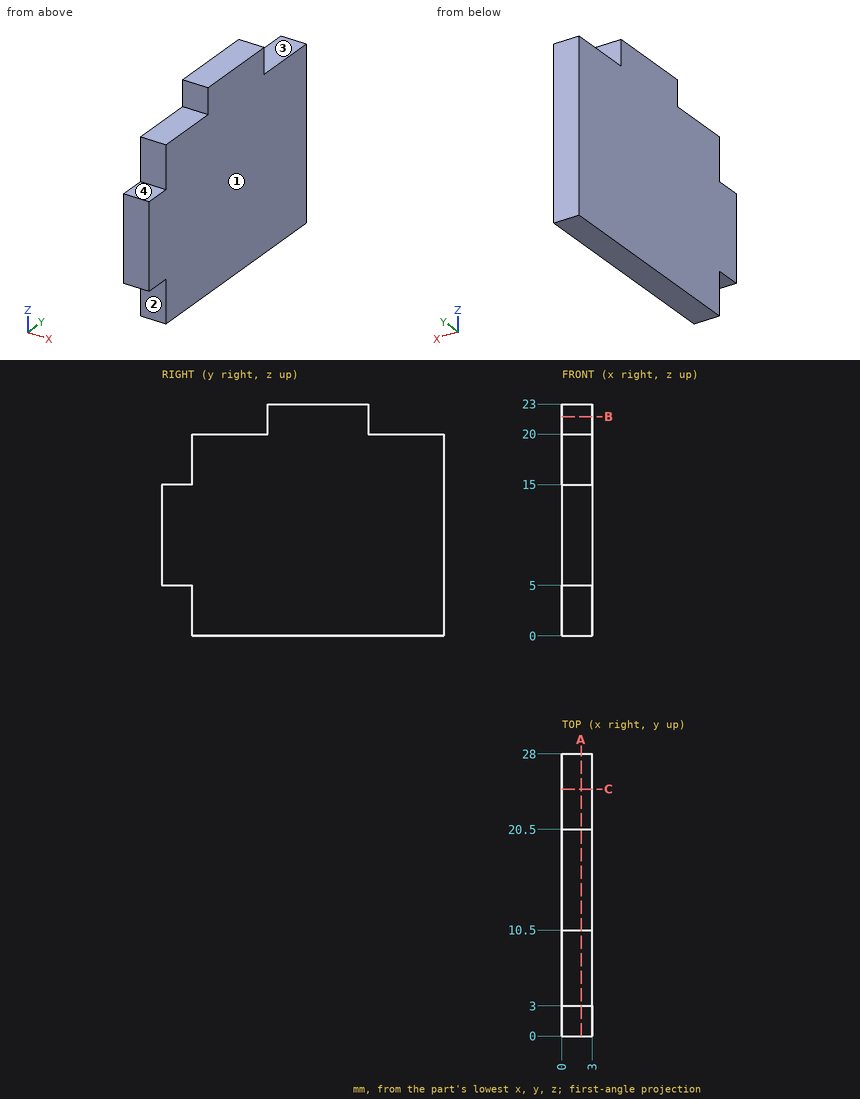
Can you work these out from the drawing? Everything is in mm from the part's minimum corner. A direction names the side the tool comes from. Round coordinates to 2 decimals unless told otherwise and drop trailing zeros. Loops run counter-clockwise (first coordinate to the right, second up) from the corner with the lowest first, then second, coordinate; pieces in that order, holes last. Notation, with made-up numbers: (23.25, 68) - (49.25, 68) arc R25 cw to (49.25, 92) - close; hole circle Ø6 at (56.5, -22.75). An arc over 180 degrees is marked (long way). Answer in a Markdown table with one row per item. Add a question column.
(1) I'm going to push flat-ended pins straight in: pin 1 (1 mm diameter, centred on x = 2, y = 18.5, fed in from -Z); pin 2 (0.9 mm diameter, centred on x = 1.5, z = 22, fed in from -Y); pin 3 (1.5 mm diameter, centred on x = 1.5, y = 1.5, fed in from -Z); pin 4 (1.5 mm diameter, centred on x = 1, z = 1.5, fed in from -Y). Where does each tip first touch, or does it pass through?
(2) If we section it at A-A (x = 1.9): Please give me the cut outline in (y, z).
(3) For the marked faces 1, 2, 3 and 4, which set-ups out of +Z, -Z, +X, -X, +Y, -Y let a thin tool reach every point of the face, with its end or its side?
(4) If we section it at C-C (y = 24.5): Please give me the cut outline in (x, z), plus the area to 3 significant figures.
(5) I need wall thicknesses on line 1 along Z through (x, y) = (1.7, 4.5); line 2 along Z through (x, y) = (1.1, 2.5); line 3 along Y through (x, z) = (2.2, 4.5). Which ranges of each line are inside material? Lowest first, please.
(6) If we section it at B-B (z = 21.75): Please give me the cut outline in (x, y), plus the area to 3 significant figures.
Model answer:
| question | item | result |
|---|---|---|
| 1 | pin 1 | stops at z = 0 |
| 1 | pin 2 | stops at y = 10.5 |
| 1 | pin 3 | stops at z = 5 |
| 1 | pin 4 | stops at y = 3 |
| 2 | outline | (0, 5) - (3, 5) - (3, 0) - (28, 0) - (28, 20) - (20.5, 20) - (20.5, 23) - (10.5, 23) - (10.5, 20) - (3, 20) - (3, 15) - (0, 15) - close |
| 3 | face 1 | +Z, -Z, +X, +Y, -Y |
| 3 | face 2 | -Z, +X, -X, -Y |
| 3 | face 3 | +Z, +X, -X, +Y |
| 3 | face 4 | +Z, +X, -X, -Y |
| 4 | outline | (0, 0) - (3, 0) - (3, 20) - (0, 20) - close |
| 4 | area | 60.0 mm² |
| 5 | line 1 | z = 0 to 20 |
| 5 | line 2 | z = 5 to 15 |
| 5 | line 3 | y = 3 to 28 |
| 6 | outline | (0, 10.5) - (3, 10.5) - (3, 20.5) - (0, 20.5) - close |
| 6 | area | 30.0 mm² |
